Input: part model. Units: mm. Frame: model coordinates. Coordinates: 2 decimals unless noted, no trailing zeros. Order: outer loops, then holes, each group sorted by start corner. A loop starts at its lowest first (then second) coordinate and runs counter-clockwise, first axis right, second up. Notation, with made-up numbers: (-15, -5.75) - (28, -5.75) arc R8 cw to (28, 9.25) - close; hole circle Ø8 at (65, 39). An arc over 180 degrees is marked (long way). Answer as CSV lines item,"result". Start each with the question number.
Item 1: First-contact query: pin 1 (14 mm diameter, centred on x = 120.65, z = -88.9, fed in from -Y). Flat tip, straight axial feed; report the tip coordinate or a pass-through.
Item 2: Section D-D (y = 0.8). Output: boundary loops of the cut face in (x, z).
Item 3: Section B-B (z = -103.5). Output: boundary loops of the cut face in (x, y).
Item 4: Section C-C (x = 120.65). Output: boundary loops of the cut face in (y, z), and give its area (3 significant figures).
Item 5: Section A-A (z = -88.9). Output: boundary loops of the cut face in (x, y).
Item 6: Draft query along Z for faces 1 (the cylindrical face through (124.341, 1.252, -92.925)), 2 (the flat face through (95, 2.54, -73)). Return one class per face: +Z half, -Z half, draft (parallel to the pull), parting line (faces both ways), or undercut.
Item 7: Material intervals for line 1 along X through (y, z) = (1.15, -88.9); line 2 along Z through (x, y) = (161, 0.8); line 3 along X through (y, z) = (0.9, -93), sorted ascending.
from build123d import *

# Parameters (mm, degrees)
SKETCH1_W           = 191.77
SKETCH1_H           = 144.78
SKETCH1_R           = 5.461
SKETCH1_W_2         = 25.908
SKETCH1_H_2         = 32.2834
BOSS_EXTRUDE1_DEPTH = 2.54


with BuildPart() as part:
    # Sketch1 → Boss-Extrude1 (new body)
    with BuildSketch(Plane(origin=(0, 0, 0), x_dir=(1, 0, 0), z_dir=(0, 1, 0))):
        with Locations((95.885, 72.39)):
            Rectangle(SKETCH1_W, SKETCH1_H)
        with Locations(Location((120.65, 88.9, 0), (0, 0, 270))):  # turned: the seam where the file's is
            Circle(SKETCH1_R, mode=Mode.SUBTRACT)
        with Locations((153.416, 95.6183)):
            Rectangle(SKETCH1_W_2, SKETCH1_H_2, mode=Mode.SUBTRACT)
    extrude(amount=BOSS_EXTRUDE1_DEPTH)


solid = part.part
Determined:
1,pin 1,"stops at y = 0"
2,outline,"(0, -144.78) - (191.77, -144.78) - (191.77, 0) - (0, 0) - close; hole circle Ø10.92 at (120.65, -88.9); hole (140.46, -111.76) - (166.37, -111.76) - (166.37, -79.48) - (140.46, -79.48) - close"
3,outline,"(0, 0) - (140.46, 0) - (140.46, 2.54) - (0, 2.54) - close; (166.37, 0) - (191.77, 0) - (191.77, 2.54) - (166.37, 2.54) - close"
4,outline,"(0, -144.78) - (2.54, -144.78) - (2.54, -94.36) - (0, -94.36) - close; (0, -83.44) - (2.54, -83.44) - (2.54, 0) - (0, 0) - close"
4,area,"340 mm^2"
5,outline,"(0, 0) - (115.19, 0) - (115.19, 2.54) - (0, 2.54) - close; (126.11, 0) - (140.46, 0) - (140.46, 2.54) - (126.11, 2.54) - close; (166.37, 0) - (191.77, 0) - (191.77, 2.54) - (166.37, 2.54) - close"
6,face 1,"undercut"
6,face 2,"draft"
7,line 1,"x = 0 to 115.19, 126.11 to 140.46, 166.37 to 191.77"
7,line 2,"z = -144.78 to -111.76, -79.48 to 0"
7,line 3,"x = 0 to 117.04, 124.26 to 140.46, 166.37 to 191.77"
